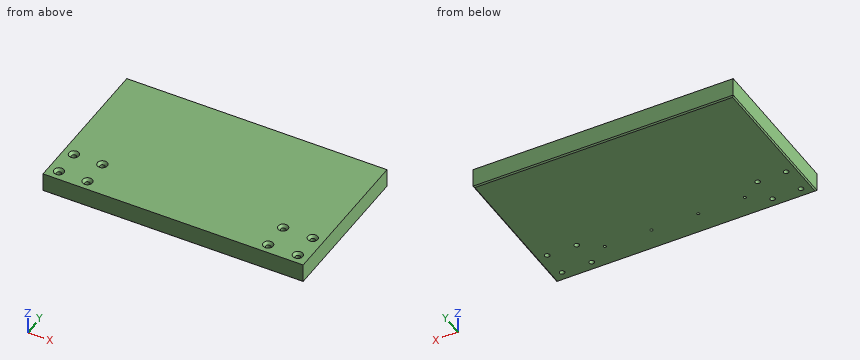
from build123d import *

# Parameters (mm, degrees)
SKETCH2_W               = 334.5
SKETCH2_H               = 194.1
PRIMARY_EXTRUSION_DEPTH = 25.4
RAIL_START              = -25.4
RAIL_MOUNTING_DEPTH     = 10
SKETCH3_R               = 3.175
CUT_EXTRUDE2_DEPTH      = 26.4
CHAMFER1_SIZE           = 3.175
CHAMFER2_SIZE           = 1.5875


with BuildPart() as part:
    # Sketch2 → Primary Extrusion (new body)
    with BuildSketch(Plane.XY):
        with Locations((-21.625, 97.05)):
            Rectangle(SKETCH2_W, SKETCH2_H)
    extrude(amount=-PRIMARY_EXTRUSION_DEPTH)

    # Sketch2<3> → Rail Mounting (cut)
    with BuildSketch(Plane.XY.offset(RAIL_START)):
        with BuildLine():
            ThreePointArc((-112.875, 31.75), (-114.625, 30), (-112.875, 28.25))
            ThreePointArc((-112.875, 28.25), (-111.125, 30), (-112.875, 31.75))
        make_face()
        with BuildLine():
            ThreePointArc((-52.875, 31.75), (-54.625, 30), (-52.875, 28.25))
            ThreePointArc((-52.875, 28.25), (-51.125, 30), (-52.875, 31.75))
        make_face()
        with BuildLine():
            ThreePointArc((7.125, 31.75), (5.375, 30), (7.125, 28.25))
            ThreePointArc((7.125, 28.25), (8.875, 30), (7.125, 31.75))
        make_face()
        with BuildLine():
            ThreePointArc((67.125, 31.75), (65.375, 30), (67.125, 28.25))
            ThreePointArc((67.125, 28.25), (68.875, 30), (67.125, 31.75))
        make_face()
    extrude(amount=RAIL_MOUNTING_DEPTH, mode=Mode.SUBTRACT)

    # Sketch3 → Cut-Extrude2 (cut, through all)
    with BuildSketch(Plane.XY):
        with Locations((-138.815833333, 47.3)):
            Circle(SKETCH3_R)
        with Locations((-138.815833333, 12.7)):
            Circle(SKETCH3_R)
        with Locations((93.595, 47.3)):
            Circle(SKETCH3_R)
        with Locations((131.655, 47.3)):
            Circle(SKETCH3_R)
        with Locations((131.655, 12.7)):
            Circle(SKETCH3_R)
        with Locations((93.595, 12.7)):
            Circle(SKETCH3_R)
        with Locations((-175.434166667, 12.7)):
            Circle(SKETCH3_R)
        with Locations((-175.434166667, 47.3)):
            Circle(SKETCH3_R)
    extrude(amount=-CUT_EXTRUDE2_DEPTH, mode=Mode.SUBTRACT)

    # Chamfer1
    chamfer1_edges = [part.edges().sort_by_distance(p)[0] for p in [
        (128.48, 12.7, 0),
        (90.42, 47.3, 0),
        (128.48, 47.3, 0),
        (-141.990833333, 12.7, 0),
        (90.42, 12.7, 0),
        (-178.609166667, 12.7, 0),
        (-178.609166667, 47.3, 0),
        (-141.990833333, 47.3, 0),
    ]]
    chamfer(chamfer1_edges, length=CHAMFER1_SIZE)

    # Chamfer2
    chamfer2_edges = [part.edges().sort_by_distance(p)[0] for p in [
        (-21.625, 0, -25.4),
        (145.625, 97.05, -25.4),
        (-21.625, 194.1, -25.4),
        (-188.875, 97.05, -25.4),
    ]]
    chamfer(chamfer2_edges, length=CHAMFER2_SIZE)


solid = part.part
CAD build for the part. Positions are in the model's coordinates, mm. Coordinates: 2 decimals unless noted, no trailing zeros. Write item = value, one per line. Start each with the question number.
Q1. Flat gauge pins, fed straight in: pin 1 Ø3 at (x, y) = (68, 30) entering from -Z; pin 2 Ø1 at (x, y) = (7.5, 30.5) entering from -Z; pin 3 Ø10 at (x, y) = (-138.82, 12.7) entering from +Z. Where does each tip first touch, or does it go through?
Q2. Drill centre lines: L1, parallel to X at y = 30, z = -20 (3 decimals); L2, parallel to Y at x = 129, z = -19.75. Where is each one in solid material? Low to high.
Q3. Cut at A-A, the plane y = 12.7. Give the number of separate pieces and of enclosed holes in the cut face, then the cut area to 3 significant figures.
Computed:
q1.pin_1 = -25.4
q1.pin_2 = -15.4
q1.pin_3 = -1.35
q2.L1 = -188.875 to -114.625, -111.125 to -54.625, -51.125 to 5.375, 8.875 to 65.375, 68.875 to 145.625
q2.L2 = 0 to 10.96, 14.44 to 45.56, 49.04 to 194.1
q3.separate_pieces = 5
q3.enclosed_holes = 0
q3.area = 7,810 mm²
